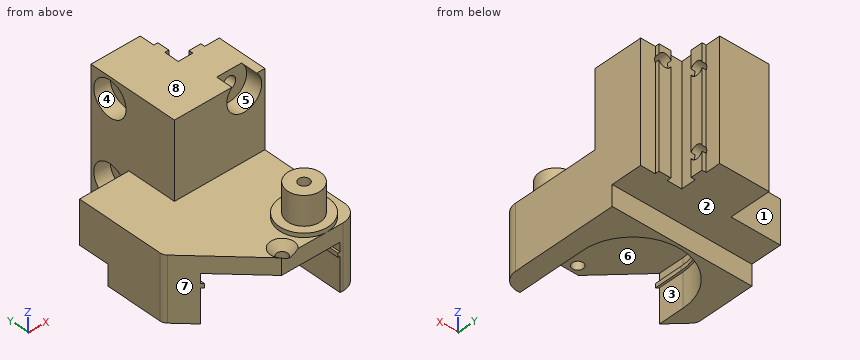
```python
from build123d import *

# Parameters (mm, degrees)
BASE_SKETCHUP_W                   = 34
BASE_SKETCHUP_H                   = 37
BASE_EXTRUSION_DEPTH              = 15.5
FIX_EXTRUSION_DEPTH               = 34
BALL_EXTRUSION_DEPTH              = 29
BALL_BEARING_BASE_SKETCHUP_R      = 6
BALL_BEARING_BASE_EXTRUSION_DEPTH = 1
BALL_BEARING_SKETCHUP_R           = 4
BALL_BEARING_EXTRUSION_DEPTH      = 7
BALL_BEARING_FIX_SKETCHUP_R       = 1.3
BALL_BEARING_FIX_HOLE_DEPTH       = 12
BOSS_EXTRU_5_DEPTH                = 11.5
BOSS_EXTRU_6_DEPTH                = 1
ESQUISSE13_W                      = 5
ESQUISSE13_H                      = 17.5
ENL_V_MAT_EXTRU_1_DEPTH           = 35
CONG_2_R                          = 4
ENL_V_MAT_EXTRU_2_DEPTH           = 16.5
CONG_4_R                          = 2
ESQUISSE16_R                      = 1.6
MAKERBEAMINTERIORHOLES1_DEPTH     = 23
ESQUISSE17_R                      = 4.25
MAKERBEAMINTERIORHOLES2_DEPTH     = 4
ESQUISSE18_R                      = 1.6
MAKERBEAMFRONTHOLE1_DEPTH         = 23
ESQUISSE19_R                      = 4.25
MAKERBEAMFRONTHOLE2_DEPTH         = 4
ESQUISSE20_W                      = 37
ESQUISSE20_H                      = 47
ENL_V_MAT_EXTRU_7_DEPTH           = 35


with BuildPart() as part:
    # Base Sketchup → Base Extrusion (new body)
    with BuildSketch(Plane.XY):
        Rectangle(BASE_SKETCHUP_W, BASE_SKETCHUP_H)
    extrude(amount=BASE_EXTRUSION_DEPTH)


with BuildPart() as body_2:
    # Fix Sketchup → Fix Extrusion (new body)
    with BuildSketch(Plane(origin=(0, 0, 0), x_dir=(-1, 0, 0), z_dir=(0, 0, -1))):
        Polygon((17, 18.5), (13.45, 18.5), (13.45, 19.5), (10.55, 19.5), (10.55, 18.5), (7, 18.5), (7, 22.05), (8, 22.05), (8, 24.95), (7, 24.95), (7, 28.5), (-5, 28.5), (-5, 6.5), (17, 6.5), align=None)
    extrude(amount=-FIX_EXTRUSION_DEPTH)


with BuildPart() as ball_extrusion_tool:
    # Ball Place Sketchup → Ball Extrusion (new body)
    with BuildSketch(Plane.XZ.offset(18.5)):
        Polygon((-12.25, 0), (-12.25, 8.25), (-11.75, 8.25), (-11.75, 9.25), (-12.25, 9.25), (-12.25, 11.5), (12.25, 11.5), (12.25, 9.25), (11.75, 9.25), (11.75, 8.25), (12.25, 8.25), (12.25, 0), align=None)
    extrude(amount=-BALL_EXTRUSION_DEPTH)


with BuildPart() as part_1:
    add(part.part)

    # Ball Extrusion: cut by ball_extrusion_tool
    add(ball_extrusion_tool.part, mode=Mode.SUBTRACT)

    # Esquisse12 → Fraisage pour vis à tête fraisée bombée #41 (revolve, cut)
    with BuildSketch(Plane(origin=(0, -16.5, 15.5), x_dir=(0, -1, 0), z_dir=(1, 0, 0))):
        Polygon((0, 0), (0, 15.5), (1.3, 15.5), (1.3, 1.791698794), (2.8575, 0), align=None)
    revolve(axis=Axis((0, -16.5, 21.85), (0, 0, -1)), mode=Mode.SUBTRACT)

    # Ball Bearing Base Sketchup → Ball Bearing Base Extrusion (add)
    with BuildSketch(Plane.XY.offset(15.5)):
        with Locations((-9, -12.5)):
            Circle(BALL_BEARING_BASE_SKETCHUP_R)
    extrude(amount=BALL_BEARING_BASE_EXTRUSION_DEPTH)

    # Ball Bearing Sketchup → Ball Bearing Extrusion (add)
    with BuildSketch(Plane.XY.offset(16.5)):
        with Locations((-9, -12.5)):
            Circle(BALL_BEARING_SKETCHUP_R)
    extrude(amount=BALL_BEARING_EXTRUSION_DEPTH)

    # Ball Bearing Fix Sketchup → Ball Bearing Fix Hole (cut)
    with BuildSketch(Plane.XY.offset(23.5)):
        with Locations((-9, -12.5)):
            Circle(BALL_BEARING_FIX_SKETCHUP_R)
    extrude(amount=-BALL_BEARING_FIX_HOLE_DEPTH, mode=Mode.SUBTRACT)



with BuildPart() as body_2_1:
    add(body_2.part)

    # Ball Extrusion: cut by ball_extrusion_tool
    add(ball_extrusion_tool.part, mode=Mode.SUBTRACT)


with BuildPart() as part_2:
    add(part_1.part)

    add(body_2_1.part)  # Boss.-Extru.5 merges body 2
    # Esquisse10 → Boss.-Extru.5 (add)
    with BuildSketch(Plane(origin=(0, 0, 11.5), x_dir=(-1, 0, 0), z_dir=(0, 0, -1))):
        with BuildLine():
            Line((12.25, -2), (12.25, 10.5))
            Line((12.25, 10.5), (-12.25, 10.5))
            Line((-12.25, 10.5), (-12.25, -2))
            ThreePointArc((-12.25, -2), (0, 10.25), (12.25, -2))
        make_face()
    extrude(amount=BOSS_EXTRU_5_DEPTH)

    # Esquisse11 → Boss.-Extru.6 (add)
    with BuildSketch(Plane(origin=(0, 0, 8.25), x_dir=(-1, 0, 0), z_dir=(0, 0, -1))):
        with BuildLine():
            Line((11.75, -2), (12.25, -2))
            Line((12.25, -2), (12.25, 10.25))
            Line((12.25, 10.25), (-12.25, 10.25))
            Line((-12.25, 10.25), (-12.25, -2))
            Line((-12.25, -2), (-11.75, -2))
            ThreePointArc((-11.75, -2), (0, 9.75), (11.75, -2))
        make_face()
    extrude(amount=-BOSS_EXTRU_6_DEPTH)

    # Esquisse13 → Enlèv. mat.-Extru.1 (cut, through all)
    with BuildSketch(Plane(origin=(17, 0, 0), x_dir=(0, 0, -1), z_dir=(1, 0, 0))):
        with Locations((-2.5, 19.75)):
            Rectangle(ESQUISSE13_W, ESQUISSE13_H)
    extrude(amount=-ENL_V_MAT_EXTRU_1_DEPTH, mode=Mode.SUBTRACT)

    # Congé2
    cong_2_edges = [part_2.edges().sort_by_distance(p)[0] for p in [
        (-17, -18.5, 7.75),
    ]]
    fillet(cong_2_edges, radius=CONG_2_R)

    # Esquisse14 → Enlèv. mat.-Extru.2 (cut, through all)
    with BuildSketch(Plane.XY.offset(15.5)):
        Polygon((2, -18.5), (17, -3.5), (17, -18.5), align=None)
    extrude(amount=-ENL_V_MAT_EXTRU_2_DEPTH, mode=Mode.SUBTRACT)

    # Congé4
    cong_4_edges = [part_2.edges().sort_by_distance(p)[0] for p in [
        (17, -3.5, 7.75),
    ]]
    fillet(cong_4_edges, radius=CONG_4_R)

    # Esquisse16 → MakerBeamInteriorHoles1 (cut, through all)
    with BuildSketch(Plane(origin=(5, 0, 0), x_dir=(0, 0, -1), z_dir=(1, 0, 0))):
        with Locations((-29, 23.5)):
            Circle(ESQUISSE16_R)
        with Locations((-10, 23.5)):
            Circle(ESQUISSE16_R)
    extrude(amount=-MAKERBEAMINTERIORHOLES1_DEPTH, mode=Mode.SUBTRACT)

    # Esquisse17 → MakerBeamInteriorHoles2 (cut)
    with BuildSketch(Plane(origin=(5, 0, 0), x_dir=(0, 0, -1), z_dir=(1, 0, 0))):
        with Locations((-29, 23.5)):
            Circle(ESQUISSE17_R)
        with Locations((-10, 23.5)):
            Circle(ESQUISSE17_R)
    extrude(amount=-MAKERBEAMINTERIORHOLES2_DEPTH, mode=Mode.SUBTRACT)

    # Esquisse18 → MakerBeamFrontHole1 (cut, through all)
    with BuildSketch(Plane(origin=(0, 6.5, 0), x_dir=(-1, 0, 0), z_dir=(0, -1, 0))):
        with Locations((12, -31)):
            Circle(ESQUISSE18_R)
    extrude(amount=-MAKERBEAMFRONTHOLE1_DEPTH, mode=Mode.SUBTRACT)

    # Esquisse19 → MakerBeamFrontHole2 (cut)
    with BuildSketch(Plane(origin=(0, 6.5, 0), x_dir=(-1, 0, 0), z_dir=(0, -1, 0))):
        with Locations((12, -31)):
            Circle(ESQUISSE19_R)
    extrude(amount=-MAKERBEAMFRONTHOLE2_DEPTH, mode=Mode.SUBTRACT)


with BuildPart() as body_2_2:
    # Symétrie2: mirrored copy
    add(part_2.part.mirror(Plane(origin=(20, 0, 0), x_dir=(0, 0, 1), z_dir=(1, 0, 0))))


with BuildPart() as part_3:
    add(part_2.part)

    # Esquisse20 → Enlèv. mat.-Extru.7 (cut, through all)
    with BuildSketch(Plane.XY.offset(34)):
        with Locations((1.5, 5)):
            Rectangle(ESQUISSE20_W, ESQUISSE20_H)
    extrude(amount=-ENL_V_MAT_EXTRU_7_DEPTH, mode=Mode.SUBTRACT)


solid = body_2_2.part
```
Check sheet for the modelled part. Datum: model origin and axes. Units: mm. Face numbers are marked on the shaded views. A direction names the side the tool comes from. Round coordinates to 2 decimals unless told otherwise and drop trailing zeros. Order: outer loops, then holes, each group sorted by start corner. A loop starts at its lowest first (then second) coordinate and runs counter-clockwise, first axis right, second up. Notation, with made-up numbers: (-26, 58) - (-6, 58) arc R23 cw to (-6, 96) - close; hole circle Ø7 at (-19.75, 37). An arc over 180 degrees is marked (long way). Answer as CSV lines item,"result". Start each with the question number.
1) Tool access check on the marked faces 1, 2, 3, 4 and 5. Record the directions out of +Z, -Z, +X, -X, +Y, -Y that give a thin tool (end or side, any length) a straight path to the whole face; none if there is none.
2) Section check C-C (x = 31.5). Record the cut outline in (y, z).
3) Draft check along X on the marked faces 6, 7 and 8. Enter one of: +X half, -X half, draft (parallel to the pull), parting line (faces both ways), or undercut.
4) Depth check by flat-ended pin: pin 1 (6.5 mm diameter, centred on y = -8.5, z = 3.5, fed in from -X); pin 2 (9 mm diameter, centred on x = 32.5, y = 22, fed in from -Z); pin 3 (10 mm diameter, centred on x = 43, z = 23, fed in from -Y). Enter the tip coordinate at first touch or a pass-through.
5) Section check B-B (z = 4). Record the cut outline in (x, y).
6) Section check D-D (y = -7.5). Record the cut outline in (x, z).
7) Scan lines: probe 1 along X at (y, z) = (19, 15); probe 2 along Y at (x, z) = (36, 29); probe 3 along Y at (x, z) = (40, 12.4). Record each from-to range of solid material in increasing order.
8) Section check A-A (y = 23.5). Record the cut outline in (x, z), then the cut area to 3 significant figures.
Determined:
1,face 1,"+Z, -Z, -X, +Y"
1,face 2,"-Z, +X, -X, +Y"
1,face 3,"-Z, -Y"
1,face 4,"-X"
1,face 5,"-Y"
2,outline,"(-12, 11.5) - (6.82, 11.5) - (6.82, 9.25) - (6.11, 9.25) - (6.11, 8.25) - (6.82, 8.25) - (6.82, 0) - (11, 0) - (11, 5) - (18.5, 5) - (18.5, 15.5) - (-12, 15.5) - close"
3,face 6,"undercut"
3,face 7,"-X half"
3,face 8,"draft"
4,pin 1,"x = 24.75"
4,pin 2,"z = 5"
4,pin 3,"y = -16.37"
5,outline,"(23, -2.67) arc R2 ccw to (23.59, -4.09) - (27.75, -8.25) - (27.75, -2) arc R12.25 cw to (52.25, -2) - (52.25, -18.5) - (53, -18.5) arc R4 ccw to (57, -14.5) - (57, 11) - (23, 11) - close"
6,outline,"(27, 0) - (27.75, 0) - (27.75, 8.25) - (28.25, 8.25) - (28.25, 9.25) - (27.75, 9.25) - (27.75, 11.5) - (52.25, 11.5) - (52.25, 9.25) - (51.75, 9.25) - (51.75, 8.25) - (52.25, 8.25) - (52.25, 0) - (57, 0) - (57, 15.5) - (52.32, 15.5) - (52.32, 16.5) - (45.68, 16.5) - (45.68, 15.5) - (27, 15.5) - close"
7,probe 1,"35 to 47, 50.55 to 53.45"
7,probe 2,"6.5 to 19.25, 27.75 to 28.5"
7,probe 3,"-18.5 to -17.8, -15.2 to 28.5"
8,outline,"(35, 5) - (48, 5) - (48, 8.4) - (39, 8.4) - (39, 5.75) - (35, 5.75) - close; (35, 14.25) - (39, 14.25) - (39, 11.6) - (48, 11.6) - (48, 27.4) - (39, 27.4) - (39, 24.75) - (35, 24.75) - close; (35, 33.25) - (39, 33.25) - (39, 30.6) - (48, 30.6) - (48, 34) - (35, 34) - close"
8,area,"251 mm^2"
